Geometry: see drawing. Coordinates: mm, zero at the bounding-box minimum. Coordinates: 2 decimals unless noted, no trailing zeros. Write each loop counter-clockwise with the first axis right and the second up, starting at its lowest first coordinate (ties: lowest second). Pieces come first, ordered by that corner, then holes. Notation, with made-up numbers: M 87,8 L 92,8 A28 cw 92,44 Z; hole C 8,17 d3. An arc over 180 degrees is marked long. One line per item, written item: value. Start each with the question number.
Item 1: Cut plane C-C, the plane x = 9.75. Output: boundary loops of the cut face in (y, z).
Item 2: Cut plane B-B, the plane z = 48. Output: boundary loops of the cut face in (x, y).
Item 3: Ray query, L1, parallel to Y at x = 3.5, z = 41.5; L2, parallel to Y at x = 8.25, z = 46.5; L3, parallel to Z at x = 0.75, y = 71.5 (1 decimal). Return the intervals inside material, ascending. Write a range as from..to.
Item 4: Cut plane D-D, the plane x = 2.75. Output: boundary loops of the cut face in (y, z).
Item 5: Pin query (flat end, axial travel): P1, Ø5, axis at x = 5.5, y = 111, coming from the +Z side; P2, Ø5, axis at x = 8.5, y = 43, coming from the +Z side; P3, Ø5, axis at x = 3, y = 45.5, coming from the +Z side. Return the tip coordinate at first contact, or that it passes through.
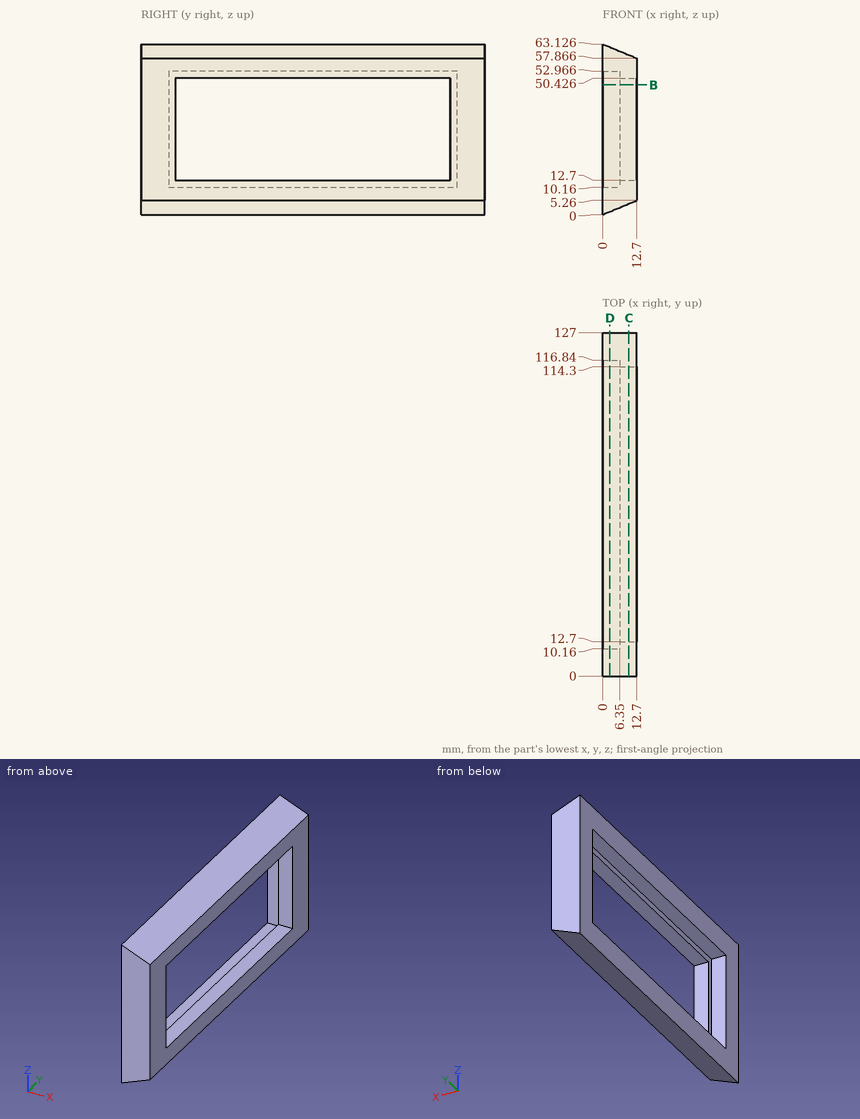
From the geometry:
1. outline: M 0,4.04 L 127,4.04 L 127,59.09 L 0,59.09 Z; hole M 12.7,12.7 L 114.3,12.7 L 114.3,50.43 L 12.7,50.43 Z
2. outline: M 0,0 L 12.7,0 L 12.7,12.7 L 6.35,12.7 L 6.35,10.16 L 0,10.16 Z; M 0,116.84 L 6.35,116.84 L 6.35,114.3 L 12.7,114.3 L 12.7,127 L 0,127 Z
3. L1: y = 0..10.16, 116.84..127
3. L2: y = 0..12.7, 114.3..127
3. L3: z = 0.3..10.2, 53..62.8
4. outline: M 0,1.14 L 127,1.14 L 127,61.99 L 0,61.99 Z; hole M 10.16,10.16 L 116.84,10.16 L 116.84,52.97 L 10.16,52.97 Z
5. P1: stops at z = 61.88
5. P2: stops at z = 60.64
5. P3: stops at z = 62.92
